from build123d import *

# Parameters (mm, degrees)
SKETCH1_W           = 60
SKETCH1_H           = 42
SKETCH1_W_2         = 56
SKETCH1_H_2         = 38
BOSS_EXTRUDE1_DEPTH = 50
SKETCH2_W           = 42
SKETCH2_H           = 95
BOSS_EXTRUDE2_DEPTH = 3
SKETCH3_R           = 12.5
CUT_EXTRUDE1_DEPTH  = 3


with BuildPart() as part:
    # Sketch1 → Boss-Extrude1 (new body)
    with BuildSketch(Plane(origin=(0, 0, 0), x_dir=(1, 0, 0), z_dir=(0, 1, 0))):
        Rectangle(SKETCH1_W, SKETCH1_H)
        Rectangle(SKETCH1_W_2, SKETCH1_H_2, mode=Mode.SUBTRACT)
    extrude(amount=BOSS_EXTRUDE1_DEPTH)

    # Sketch2 → Boss-Extrude2 (add)
    with BuildSketch(Plane(origin=(30, 0, 0), x_dir=(0, 0, -1), z_dir=(1, 0, 0))):
        with Locations((0, 47.5)):
            Rectangle(SKETCH2_W, SKETCH2_H)
    extrude(amount=BOSS_EXTRUDE2_DEPTH)

    # Sketch3 → Cut-Extrude1 (cut)
    with BuildSketch(Plane(origin=(33, 0, 0), x_dir=(0, 0, -1), z_dir=(1, 0, 0))):
        with Locations((0, 71)):
            Circle(SKETCH3_R)
    extrude(amount=-CUT_EXTRUDE1_DEPTH, mode=Mode.SUBTRACT)


solid = part.part
Design review of the part built by this model. Coordinates are the model's own, in mm. A direction names the side the tool comes from. Round coordinates to 2 decimals unless told otherwise and drop trailing zeros. Write each loop counter-clockwise with the first axis right and the second up, starting at its lowest first coordinate (ties: lowest second). Pieces come first, ordered by that corner, then holes. Notation, with made-up numbers: (47.5, 0) - (83.5, 0) arc R29 ccw to (83.5, 37) - close; hole circle Ø9 at (58.25, 72.25). An arc over 180 degrees is marked (long way). Return JSON: item names as keys, results as strings. Group by question number.
Item 1: We need section A-A on z = 0. Write out the cut boundary in (x, y).
Item 2: We need section C-C on y = 71. Write out the cut boundary in (x, z), and give its area (3 significant figures).
Item 3: The part is to be moulded in two halves that separate along X. For faces 1 (the face through (0, 25, 19)), 2 (the face through (33, 48, 0)), 3 (the face through (8, 0, 20)), say which applies: pulls with the +X half, pulls with the -X half, needs draft (parallel to the pull), parting line crosses it, or undercut.
Item 4: We need section B-B on z = 16.5. Write out the cut boundary in (x, y), and give its area (3 significant figures).
Item 5: Machinability: for faces 4 (the face through (1, 26, 21)), 5 (the face through (-2, 50, 20)), 6 (the face through (0, 25, -19)), which of the approach directions +Z, -Z, +X, -X, +Y, -Y give a long, thin tool a straight path to every point of the face, cutting with its end or side? Answer none if there is none.
Item 6: Insertion check: P1, Ø12.5, axis at y = 79, z = -9.5, coming from the -X side. The pin has a flat end and moves straight along its axis. Give the tip position at first contact, or say it passes through.
Item 7: For probe 1 along X at (y, z) = (36, -12); probe 2 along Z at (x, y) = (24, 12.5); probe 3 along Y at (x, z) = (31.05, 0), list the stretches that pass through material, from the lowest coordinate up. Write a range as [from, to].
Item 8: We need section D-D on x = 11.5. Write out the cut boundary in (y, z).
Model answer:
{
 "1": {"outline": "(-30, 0) - (-28, 0) - (-28, 50) - (-30, 50) - close; (28, 0) - (33, 0) - (33, 58.5) - (30, 58.5) - (30, 50) - (28, 50) - close; (30, 83.5) - (33, 83.5) - (33, 95) - (30, 95) - close"},
 "2": {"outline": "(30, -21) - (33, -21) - (33, -12.5) - (30, -12.5) - close; (30, 12.5) - (33, 12.5) - (33, 21) - (30, 21) - close", "area": "51.0 mm²"},
 "3": {"face 1": "undercut", "face 2": "pulls with the +X half", "face 3": "needs draft"},
 "4": {"outline": "(-30, 0) - (-28, 0) - (-28, 50) - (-30, 50) - close; (28, 0) - (33, 0) - (33, 95) - (30, 95) - (30, 50) - (28, 50) - close", "area": "485 mm²"},
 "5": {"face 4": "+Z, +X, -X, +Y, -Y", "face 5": "+Z, -Z, -X, +Y", "face 6": "+Y, -Y"},
 "6": {"P1": "stops at x = 30"},
 "7": {"probe 1": "x = [-30, -28], [28, 33]", "probe 2": "z = [-21, -19], [19, 21]", "probe 3": "y = [0, 58.5], [83.5, 95]"},
 "8": {"outline": "(0, -21) - (50, -21) - (50, -19) - (0, -19) - close; (0, 19) - (50, 19) - (50, 21) - (0, 21) - close"}
}
